The listing builds one solid part. Answer for the finished solid, in the listing's coordinates (mm). A direction names the side the tool comes from. Round coordinates to 2 decimals unless told otherwise and drop trailing zeros. Write each loop counter-clockwise with the first axis right and the second up, starting at its lowest first coordinate (ties: lowest second). Pieces come first, ordered by that corner, then holes.
(1) A cutting plane is placed at C-C, the plane x = -2. Give the vertices of the cut face in (y, z).
(2) A cutting plane is placed at D-D, the plane x = -10.5. Give the vertices of the cut face in (y, z), and give its area (3 significant figures).
(3) For faces 4 (the face through (-20, 2, 5.5)), 5 (the face through (-35, 2, 0)), 6 (the face through (-5, 2, 0)), 7 (the face through (-20, 2, -5.5)), determine the directions among +Z, -Z, +X, -X, +Y, -Y from which every point of the face is accessible in a straight line to the end or side of a thin tool.
(4) Each of these flat-tipped pins is pushed along its axis until it touches: pin 1 Ø0.8 at (x, y) = (-18.5, 2.5) entering from -Z; pin 2 Ø0.5 at (x, y) = (-23.5, 2) entering from +Z; pin 3 Ø2 at (x, z) = (-2, 1.33) entering from -Y. Where does it stop, or does it pass through?
(5) A cutting plane is placed at B-B, the plane y = 0.5. Give the vertices of the cut face in (x, z).
(6) Find the intervals of material crossed by probe 1 along X at (y, z) = (0.85, 4); probe 2 along X at (y, z) = (2.2, 0.75); probe 3 along Y at (x, z) = (-13, 1.25), in increasing order.
(7) The mould has two halves that part along X. Classify faces 1 (the face through (-19, 1, -6)), 2 (the face through (-38, 1, 0)), 3 (the face through (-2.03, 0.59, 4.75)): +X half, -X half, draft (parallel to the pull), parting line (faces both ways), or undercut.
(8) A cutting plane is placed at A-A, the plane z = 4. Give the vertices of the cut face in (x, y).
from build123d import *

# Parameters (mm, degrees)
SKETCH_1_W          = 38
SKETCH_1_H          = 12
EXTRUDE_1_DEPTH     = 1.2
SKETCH_2_W          = 30
SKETCH_2_H          = 11
EXTRUDE_2_DEPTH     = 2.7
SKETCH_3_R          = 0.75
CUT_EXTRUDE_2_DEPTH = 39.565399
EXTRUDE_START       = 1.2
SKETCH_4_W          = 2
SKETCH_4_H          = 10
SKETCH_4_H_2        = 1.370131764
EXTRUDE_3_DEPTH     = 2
SKETCH_5_W          = 22.18
SKETCH_5_H          = 5.38
EXTRUDE_4_DEPTH     = 0.1


with BuildPart() as part:
    # Эскиз1 → Бобышка-Вытянуть1 (new body)
    with BuildSketch(Plane(origin=(0, 0, 0), x_dir=(1, 0, 0), z_dir=(0, 1, 0))):
        with Locations((-19, 0)):
            Rectangle(SKETCH_1_W, SKETCH_1_H)
    extrude(amount=EXTRUDE_1_DEPTH)

    # Эскиз2 → Бобышка-Вытянуть2 (add)
    with BuildSketch(Plane(origin=(0, 0, 0), x_dir=(1, 0, 0), z_dir=(0, 1, 0))):
        with Locations((-20, 0)):
            Rectangle(SKETCH_2_W, SKETCH_2_H)
    extrude(amount=EXTRUDE_2_DEPTH)

    # Эскиз3 → Вырез-Вытянуть2 (cut, through all)
    with BuildSketch(Plane(origin=(0, 0, 0), x_dir=(1, 0, 0), z_dir=(0, 1, 0))):
        with Locations(Location((-2, 4, 0), (0, 0, 90))):
            Circle(SKETCH_3_R)
        with Locations(Location((-2, 1.333333333, 0), (0, 0, 90))):
            Circle(SKETCH_3_R)
        with Locations(Location((-2, -1.333333333, 0), (0, 0, 90))):
            Circle(SKETCH_3_R)
        with Locations(Location((-2, -4, 0), (0, 0, 90))):
            Circle(SKETCH_3_R)
    extrude(amount=CUT_EXTRUDE_2_DEPTH, mode=Mode.SUBTRACT)

    # Эскиз4 → Бобышка-Вытянуть3 (add)
    with BuildSketch(Plane(origin=(0, 0, 0), x_dir=(1, 0, 0), z_dir=(0, 1, 0)).offset(EXTRUDE_START)):
        with Locations((-23, 0)):
            Rectangle(SKETCH_4_W, SKETCH_4_H)
        with Locations((-16, 0)):
            Rectangle(SKETCH_4_W, SKETCH_4_H)
        with Locations((-10.327262123, 1.918184469)):
            Rectangle(SKETCH_4_W, SKETCH_4_H_2)
    extrude(amount=-EXTRUDE_3_DEPTH)

    # Эскиз5 → Бобышка-Вытянуть4 (add)
    with BuildSketch(Plane(origin=(0, 2.7, 0), x_dir=(1, 0, 0), z_dir=(0, 1, 0))):
        with Locations((-18.32, 0.21)):
            Rectangle(SKETCH_5_W, SKETCH_5_H)
    extrude(amount=EXTRUDE_4_DEPTH)


solid = part.part
Solutions:
1. outline: (0, -6) - (1.2, -6) - (1.2, -4.75) - (0, -4.75) - close; (0, -3.25) - (1.2, -3.25) - (1.2, -2.08) - (0, -2.08) - close; (0, -0.58) - (1.2, -0.58) - (1.2, 0.58) - (0, 0.58) - close; (0, 2.08) - (1.2, 2.08) - (1.2, 3.25) - (0, 3.25) - close; (0, 4.75) - (1.2, 4.75) - (1.2, 6) - (0, 6) - close
2. outline: (-0.8, -2.6) - (0, -2.6) - (0, -6) - (1.2, -6) - (1.2, -5.5) - (2.7, -5.5) - (2.7, -2.9) - (2.8, -2.9) - (2.8, 2.48) - (2.7, 2.48) - (2.7, 5.5) - (1.2, 5.5) - (1.2, 6) - (0, 6) - (0, -1.23) - (-0.8, -1.23) - close
2. area: 32.5 mm2
3. face 4: +Z, +X, -X, +Y
3. face 5: +Z, -Z, -X, +Y
3. face 6: +Z, -Z, +X, +Y
3. face 7: -Z, +X, -X, +Y
4. pin 1: stops at z = -5.5
4. pin 2: stops at z = 5.5
4. pin 3: stops at y = 0
5. outline: (-38, -6) - (0, -6) - (0, 6) - (-38, 6) - close; hole circle Ø1.5 at (-2, -4); hole circle Ø1.5 at (-2, -1.33); hole circle Ø1.5 at (-2, 1.33); hole circle Ø1.5 at (-2, 4)
6. probe 1: x = -38 to -2.75, -1.25 to 0
6. probe 2: x = -35 to -5
6. probe 3: y = 0 to 2.8
7. face 1: draft
7. face 2: -X half
7. face 3: undercut
8. outline: (-38, 0) - (-24, 0) - (-24, -0.8) - (-22, -0.8) - (-22, 0) - (-17, 0) - (-17, -0.8) - (-15, -0.8) - (-15, 0) - (-2.75, 0) - (-2.75, 1.2) - (-5, 1.2) - (-5, 2.7) - (-35, 2.7) - (-35, 1.2) - (-38, 1.2) - close; (-1.25, 0) - (0, 0) - (0, 1.2) - (-1.25, 1.2) - close
